Autodesk Inventor part; units mm, degrees
ref_plane "YZ Plane" through (0, 0, 0) normal (1, 0, 0) x (0, 1, 0)
ref_plane "XZ Plane" through (0, 0, 0) normal (0, 1, 0) x (-1, 0, 0)
ref_plane "XY Plane" through (0, 0, 0) normal (0, 0, 1) x (1, 0, 0)
sketch "スケッチ1" plane through (0, 0, 0) normal (0, 1, 0) x (-1, 0, 0)
  circle A0 centre (0, 0) radius 2
  circle A1 centre (0, 0) radius 8
  dimension "d0" = 4
  dimension "d1" = 16
extrude "押し出し1" add sketch "スケッチ1" along normal blind 5
sketch "スケッチ2" plane through (0, 5, 0) normal (0, 1, 0) x (1, 0, 0)
  circle A0 centre (0, 0) radius 2.5
  circle A1 centre (0, 0) radius 7.5
  dimension "d4" = 5
  dimension "d5" = 15
extrude "押し出し2" cut sketch "スケッチ2" against normal blind 0.1
sketch "スケッチ3" plane through (0, 0, 0) normal (0, -1, 0) x (1, 0, 0)
  circle A0 centre (0, 0) radius 2.5
  circle A1 centre (0, 0) radius 7.5
  dimension "d8" = 5
  dimension "d9" = 15
extrude "押し出し3" cut sketch "スケッチ3" against normal blind 0.1
properties part number "Bearing_634zz" material "鋼、炭素鋼"
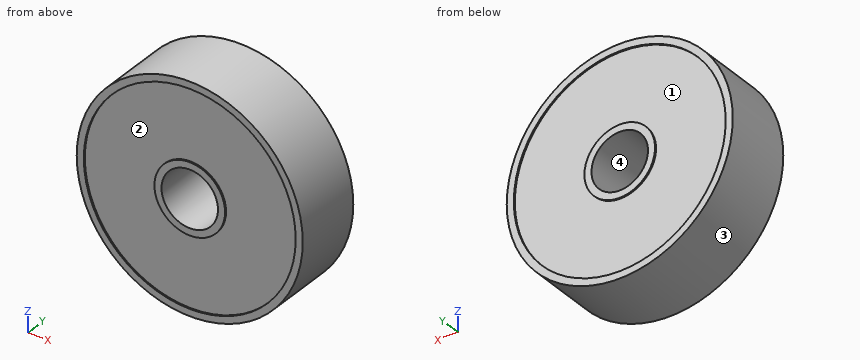
CAD build for the part. Positions are in the model's coordinates, mm. Face numbers are marked on the shaded views. A direction names the side the tool comes from. Round coordinates to 2 decimals unless told otherwise and drop trailing zeros. Order: outer loops, then holes, each group sorted by start corner. A loop starts at its lowest first (then second) coordinate and runs counter-clockwise, first axis right, second up.
Q1. Slice it at D-D (x = 5). Write the cut outline in (y, z) (3 decimals), and give its area (3 significant figures).
Q2. Slice it at B-B (z = 0.5). Write the cut outline in (x, y), and give its area (3 significant figures).
Q3. Drop flat-ended pins along their axis: pin 1 (2 mm diameter, centred on y = 4, z = 5.5, fed in from -X); pin 2 (3.5 mm diameter, centred on x = 0, z = 0, fed in from +Y). Give the stop position or say it passes through.
Q4. Which spindle directions (+Z, -Z, +X, -X, +Y, -Y) get a long thin tool onto all of the face, cutting with end or side? Do the marked faces 1 and 2. Say none if no direction does.
Q5. Slice it at C-C (y = 0.6). Write the cut outline in (x, z).
Q6. Two-plate mould, pull along Z, no slides. Class the marked faces 3 and 4: pulls with the +Z half, pulls with the -Z half, needs draft (parallel to the pull), parting line crosses it, or undercut.
Q7. Slice it at A-A (x = 0). Write the cut outline in (y, z), and give its area (3 significant figures).
Q8. Wall check: L1, parallel to Z at x = 0, y = 0.05; L2, parallel to Z at x = 0, y = 1.4; L3, parallel to Y at x = 2.75, z = -6.5. Give the ranges that are in metal, low to high.
Results below:
1. outline: (0, -6.245) - (5, -6.245) - (5, -5.59) - (4.9, -5.59) - (4.9, 5.59) - (5, 5.59) - (5, 6.245) - (0, 6.245) - (0, 5.59) - (0.1, 5.59) - (0.1, -5.59) - (0, -5.59) - close
1. area: 60.2 mm2
2. outline: (-7.98, 0) - (-7.48, 0) - (-7.48, 0.1) - (-2.45, 0.1) - (-2.45, 0) - (-1.94, 0) - (-1.94, 5) - (-2.45, 5) - (-2.45, 4.9) - (-7.48, 4.9) - (-7.48, 5) - (-7.98, 5) - close; (1.94, 0) - (2.45, 0) - (2.45, 0.1) - (7.48, 0.1) - (7.48, 0) - (7.98, 0) - (7.98, 5) - (7.48, 5) - (7.48, 4.9) - (2.45, 4.9) - (2.45, 5) - (1.94, 5) - close
2. area: 58.5 mm2
3. pin 1: stops at x = -6.61
3. pin 2: passes through
4. face 1: +Y
4. face 2: -Y
5. outline: circle Ø16 at (0, 0); hole circle Ø4 at (0, 0)
6. face 3: parting line crosses it
6. face 4: undercut
7. outline: (0, -8) - (5, -8) - (5, -7.5) - (4.9, -7.5) - (4.9, -2.5) - (5, -2.5) - (5, -2) - (0, -2) - (0, -2.5) - (0.1, -2.5) - (0.1, -7.5) - (0, -7.5) - close; (0, 2) - (5, 2) - (5, 2.5) - (4.9, 2.5) - (4.9, 7.5) - (5, 7.5) - (5, 8) - (0, 8) - (0, 7.5) - (0.1, 7.5) - (0.1, 2.5) - (0, 2.5) - close
7. area: 58.0 mm2
8. L1: z = -8 to -7.5, -2.5 to -2, 2 to 2.5, 7.5 to 8
8. L2: z = -8 to -2, 2 to 8
8. L3: y = 0.1 to 4.9
